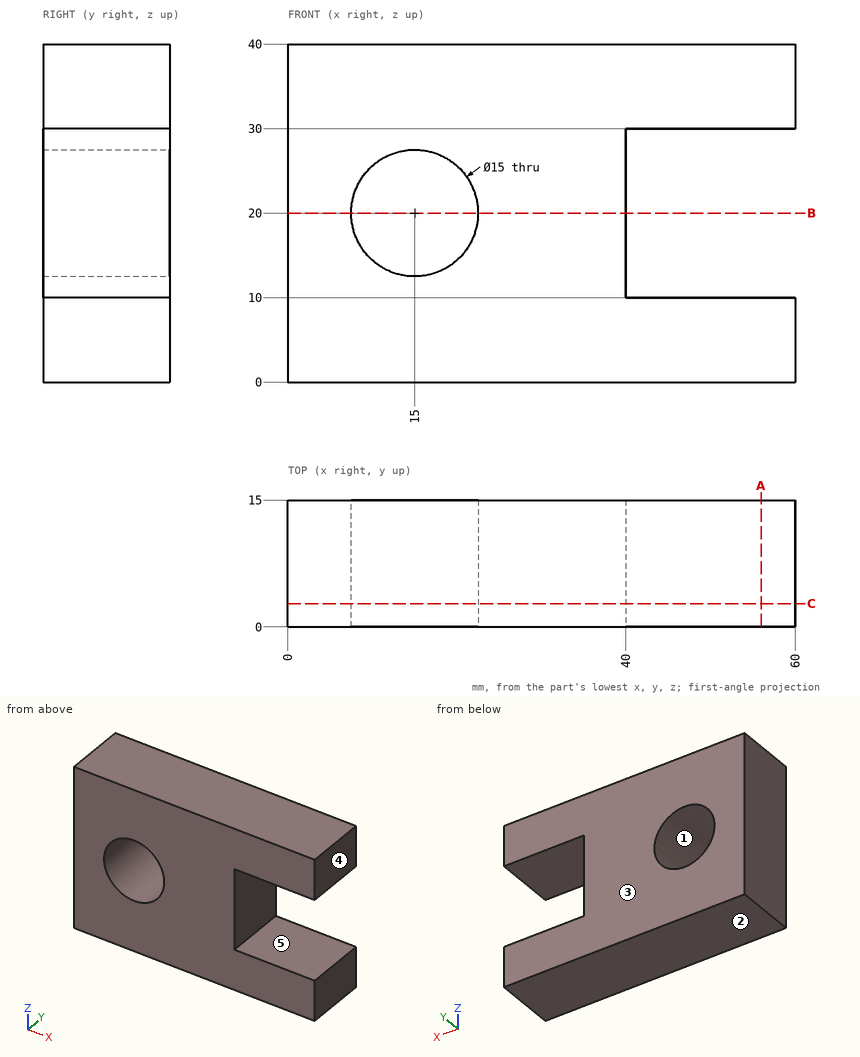
Answer from the drawing. Dimensions are ordinates in mm from the lowest x, y and z of the part. A direction names the side the tool comes from. Give positions to 0.01 mm unless a question says otherwise; leave off trailing zeros. Write each loop counter-clockwise with the first axis right and the second up, starting at its lowest first coordinate (ties: lowest second). Pieces come first, ordered by that corner, then holes. Notation, with made-up numbers: (-13, -28.75) -> (-7, -28.75) arc R13 ccw to (-7, -9.75) -> close; hole circle Ø11 at (-13.75, 87). An arc over 180 degrees is marked (long way). Use a Markdown table: item, result.
(1) For the marked faces 4 and 5, determine the directions among +Z, -Z, +X, -X, +Y, -Y from which every point of the face is accessible in a straight line to the end or side of a thin tool.
Return value:
| item | result |
|---|---|
| face 4 | +Z, -Z, +X, +Y, -Y |
| face 5 | +X, +Y, -Y |
(2) Section C-C, the plane y = 2.75 is taken. Determine the outline of the cut face in (x, z), then the cut area to 3 significant figures.
Return value:
| item | result |
|---|---|
| outline | (0, 0) -> (60, 0) -> (60, 10) -> (40, 10) -> (40, 30) -> (60, 30) -> (60, 40) -> (0, 40) -> close; hole circle Ø15 at (15, 20) |
| area | 1,820 mm2 |
(3) Find the intervals of material crossed by probe 1 along Z at (x, y) = (42, 11.75); probe 2 along X at (y, z) = (4.5, 20); probe 3 along Z at (x, y) = (15, 11), in increasing order. Write a range as from..to.
Return value:
| item | result |
|---|---|
| probe 1 | 0..10, 30..40 |
| probe 2 | 0..7.5, 22.5..40 |
| probe 3 | 0..12.5, 27.5..40 |
(4) Determine the mould class of the marked faces 1, 2 and 3 for opening direction Z: released by +Z, released by -Z, zero draft, split by the parting line, or undercut.
Return value:
| item | result |
|---|---|
| face 1 | undercut |
| face 2 | released by -Z |
| face 3 | zero draft |
(5) Section B-B, the plane z = 20 is taken. Determine the outline of the cut face in (x, y).
Return value:
| item | result |
|---|---|
| outline | (0, 0) -> (7.5, 0) -> (7.5, 15) -> (0, 15) -> close; (22.5, 0) -> (40, 0) -> (40, 15) -> (22.5, 15) -> close |
(6) Section A-A, the plane x = 56 is taken. Determine the outline of the cut face in (y, z), then the cut area to 3 significant figures.
Return value:
| item | result |
|---|---|
| outline | (0, 0) -> (15, 0) -> (15, 10) -> (0, 10) -> close; (0, 30) -> (15, 30) -> (15, 40) -> (0, 40) -> close |
| area | 300 mm2 |
